The model under review builds one solid part; all positions refer to its coordinate system, in mm. A direction names the side the tool comes from. Round coordinates to 2 decimals unless told otherwise and drop trailing zeros. Loops run counter-clockwise (first coordinate to the right, second up) from the corner with the lowest first, then second, coordinate; pieces in that order, holes last. Notation, with made-up numbers: M -28,75 L -1,75 A18 ccw -1,90 Z; hole C 84.5,-6 d4. An arc over 180 degrees is marked long. Return JSON: item names as keys, results as strings. Group by question number.
Q1. Clearance check with flat-ended pins moving along their axes: pin 1 Ø1.5 at (x, z) = (137.5, 3) entering from +Y; pin 2 Ø10 at (x, y) = (34, -17) entering from +Z; pin 3 Ø12 at (y, z) = (-47.5, 0.5) entering from -X (3 decimals); pin 4 Ø12 at (y, z) = (-40.5, -10.5) entering from +X. State where each tip first meets the part, or that it passes through.
Q2. To check wall thickness, follow line 1 along Z through (x, y) = (36.55, -75); line 2 along Y through (x, z) = (37.25, -33.5); line 3 along X through (y, z) = (-77.5, -19.5). State the ranges of each line that lie inside material, in increasing order.
Q3. Consider section A-A (z = -27). State the section outline as (x, y) points.
Q4. Draft analysis for pull direction Y (two halves, no side actions). For faces 4 (the face through (68, 13, 20)), 5 (the face through (34.52, -118.31, -1.97)), 6 (the face through (-4.8, -76.2, 11.4)), state which applies: pulls with the +Y half, pulls with the -Y half, needs draft (parallel to the pull), parting line crosses it, or undercut.
Q5. For faces 1 (the face through (34.15, -74.9, -18.5)), 2 (the face through (73.8, 4.8, 11.4)), 3 (the face through (117, -119, -4)), list the 3-axis set-ups (+Z, -Z, +X, -X, +Y, -Y) from which the entire face can be reached by the end or side of a thin tool; tool diameter is ignored.
from build123d import *

# Parameters (mm, degrees)
SHELL_2_T           = -3
SKETCH_4_R          = 1.5
CUT_EXTRUDE_1_DEPTH = 10
EXTRUDE_1_DEPTH     = 40.5
CUT_EXTRUDE_2_DEPTH = 100
SKETCH_8_R          = 1.5
EXTRUDE_2_DEPTH     = 3
EXTRUDE_3_DEPTH     = 4
EXTRUDE_4_DEPTH     = 4
SKETCH_11_W         = 56.2
SKETCH_11_H         = 25
CUT_EXTRUDE_3_DEPTH = 4


with BuildPart() as part:
    # 草图3 → 放样1 section 0
    with BuildSketch(Plane.XY.offset(20)):
        with BuildLine():
            Line((-15, 15), (165, 15))
            Line((165, 15), (165, -165))
            Line((165, -165), (-15, -165))
            Line((-15, -165), (-15, 15))
        make_face()
    # 草图1 → 放样1 section 1
    with BuildSketch(Plane.XY):
        with BuildLine():
            Line((0, 0), (150, 0))
            Line((150, 0), (150, -150))
            Line((150, -150), (0, -150))
            Line((0, -150), (0, 0))
        make_face()
    loft()

    # 抽壳2
    shell_2_openings = [part.faces().sort_by_distance(p)[0] for p in [
        (75, -75, 20),
    ]]
    offset(amount=SHELL_2_T, openings=shell_2_openings, kind=Kind.INTERSECTION)

    # 草图4 → 切除-拉伸1 (cut)
    with BuildSketch(Plane.XY.offset(3)):
        with BuildLine():
            ThreePointArc((86.25, -75), (84.75, -73.5), (83.25, -75))
            Line((83.25, -75), (86.25, -75))
        make_face()
        with BuildLine():
            Line((86.25, -75), (83.25, -75))
            ThreePointArc((83.25, -75), (84.75, -76.5), (86.25, -75))
        make_face()
        with Locations((66.25, -82)):
            Circle(SKETCH_4_R)
        with BuildLine():
            ThreePointArc((74.75, -75), (73.25, -73.5), (71.75, -75))
            Line((71.75, -75), (74.75, -75))
        make_face()
        with BuildLine():
            Line((74.75, -75), (71.75, -75))
            ThreePointArc((71.75, -75), (73.25, -76.5), (74.75, -75))
        make_face()
        with Locations((66.25, -68)):
            Circle(SKETCH_4_R)
        with BuildLine():
            ThreePointArc((60.75, -75), (59.25, -73.5), (57.75, -75))
            Line((57.75, -75), (60.75, -75))
        make_face()
        with BuildLine():
            Line((60.75, -75), (57.75, -75))
            ThreePointArc((57.75, -75), (59.25, -76.5), (60.75, -75))
        make_face()
        with BuildLine():
            ThreePointArc((49.25, -75), (47.75, -73.5), (46.25, -75))
            Line((46.25, -75), (49.25, -75))
        make_face()
        with BuildLine():
            Line((49.25, -75), (46.25, -75))
            ThreePointArc((46.25, -75), (47.75, -76.5), (49.25, -75))
        make_face()
    extrude(amount=-CUT_EXTRUDE_1_DEPTH, mode=Mode.SUBTRACT)

    # 草图6 → 凸台-拉伸1 (add)
    with BuildSketch(Plane.XY.offset(3)):
        Polygon((38.15, -62.5), (34.15, -62.5), (31.15, -62.5), (31.15, -65.5), (34.15, -65.5), (34.15, -84.5), (31.15, -84.5), (31.15, -87.5), (34.15, -87.5), (38.15, -87.5), (38.15, -75), align=None)
        Polygon((94.35, -75), (94.35, -62.5), (98.35, -62.5), (101.35, -62.5), (101.35, -65.5), (98.35, -65.5), (98.35, -84.5), (101.35, -84.5), (101.35, -87.5), (98.35, -87.5), (94.35, -87.5), align=None)
    extrude(amount=-EXTRUDE_1_DEPTH)

    # 草图7 → 切除-拉伸2 (cut)
    with BuildSketch(Plane(origin=(98.35, 0, 0), x_dir=(0, 0, -1), z_dir=(1, 0, 0))):
        with BuildLine():
            ThreePointArc((18.01, -75), (16.5, -73.49), (14.99, -75))
            Line((14.99, -75), (16.5, -75))
            Line((16.5, -75), (18.01, -75))
        make_face()
        with BuildLine():
            Line((16.5, -75), (14.99, -75))
            ThreePointArc((14.99, -75), (16.5, -76.51), (18.01, -75))
            Line((18.01, -75), (16.5, -75))
        make_face()
        with BuildLine():
            ThreePointArc((35.01, -75), (33.5, -73.49), (31.99, -75))
            Line((31.99, -75), (33.5, -75))
            Line((33.5, -75), (35.01, -75))
        make_face()
        with BuildLine():
            Line((33.5, -75), (31.99, -75))
            ThreePointArc((31.99, -75), (33.5, -76.51), (35.01, -75))
            Line((35.01, -75), (33.5, -75))
        make_face()
    extrude(amount=-CUT_EXTRUDE_2_DEPTH, mode=Mode.SUBTRACT)

    # 草图8 → 凸台-拉伸2 (add)
    with BuildSketch(Plane.XY.offset(3)):
        with Locations((66.25, -68)):
            Circle(SKETCH_8_R)
        with Locations((59.25, -75)):
            Circle(SKETCH_8_R)
        with Locations((47.75, -75)):
            Circle(SKETCH_8_R)
        with Locations((73.25, -75)):
            Circle(SKETCH_8_R)
        with Locations((84.75, -75)):
            Circle(SKETCH_8_R)
        with Locations((66.25, -82)):
            Circle(SKETCH_8_R)
    extrude(amount=-EXTRUDE_2_DEPTH)

    # 草图9 → 凸台-拉伸3 (add)
    with BuildSketch(Plane(origin=(0, 0, 0), x_dir=(-1, 0, 0), z_dir=(0, 0, -1))):
        Polygon((-73.585786438, -76.414213562), (0, -2.828427125), (0, 0), (-2.828427125, 0), (-72.748638048, -69.920210924), (-150, -147.171572875), (-150, -150), (-147.171572875, -150), align=None)
    extrude(amount=EXTRUDE_3_DEPTH)

    # 草图10 → 凸台-拉伸4 (add)
    with BuildSketch(Plane(origin=(0, 0, 0), x_dir=(-1, 0, 0), z_dir=(0, 0, -1))):
        Polygon((-106.669297814, -40.502275062), (-147.171572875, 0), (-150, 0), (-150, -2.828427125), (-121.973814525, -30.8546126), (-2.828427125, -150), (0, -150), (0, -147.171572875), align=None)
    extrude(amount=EXTRUDE_4_DEPTH)

    # 草图11 → 切除-拉伸3 (cut)
    with BuildSketch(Plane(origin=(0, 0, -4), x_dir=(-1, 0, 0), z_dir=(0, 0, -1))):
        with Locations((-66.25, -75)):
            Rectangle(SKETCH_11_W, SKETCH_11_H)
    extrude(amount=-CUT_EXTRUDE_3_DEPTH, mode=Mode.SUBTRACT)


solid = part.part
Values:
{
 "1": {"pin 1": "stops at y = 2.81", "pin 2": "stops at z = 3", "pin 3": "stops at x = -4.875", "pin 4": "passes through"},
 "2": {"line 1": "z = -37.5 to -35.01, -31.99 to -18.01, -14.99 to 3", "line 2": "y = -87.5 to -76.51, -73.49 to -62.5", "line 3": "x = 34.15 to 38.15, 94.35 to 98.35"},
 "3": {"outline": "M 31.15,-87.5 L 38.15,-87.5 L 38.15,-62.5 L 31.15,-62.5 L 31.15,-65.5 L 34.15,-65.5 L 34.15,-84.5 L 31.15,-84.5 Z; M 94.35,-87.5 L 101.35,-87.5 L 101.35,-84.5 L 98.35,-84.5 L 98.35,-65.5 L 101.35,-65.5 L 101.35,-62.5 L 94.35,-62.5 Z"},
 "4": {"face 4": "needs draft", "face 5": "pulls with the -Y half", "face 6": "undercut"},
 "5": {"face 1": "-Z, -X", "face 2": "+Z", "face 3": "-Z, +X, -X, -Y"}
}
